from build123d import *

# Parameters (mm, degrees)
SKETCH1_R           = 7.5
BOSS_EXTRUDE1_DEPTH = 35
SKETCH2_W           = 20
SKETCH2_H           = 17.5
CUT_EXTRUDE1_DEPTH  = 50
SKETCH4_R           = 15
BOSS_EXTRUDE2_DEPTH = 30
SKETCH6_R           = 9.525
CUT_EXTRUDE2_DEPTH  = 30


with BuildPart() as part:
    # Sketch1 → Boss-Extrude1 (new body)
    with BuildSketch(Plane.XY):
        with BuildLine():
            Line((-5, 12.5), (5, 12.5))
            ThreePointArc((5, 12.5), (12.071067812, 9.571067812), (15, 2.5))
            Line((15, 2.5), (15, -12.5))
            Line((15, -12.5), (-15, -12.5))
            Line((-15, -12.5), (-15, 2.5))
            ThreePointArc((-15, 2.5), (-12.071067812, 9.571067812), (-5, 12.5))
        make_face()
        with Locations((0, 2.5)):
            Circle(SKETCH1_R, mode=Mode.SUBTRACT)
    extrude(amount=BOSS_EXTRUDE1_DEPTH)

    # Sketch2 → Cut-Extrude1 (cut)
    with BuildSketch(Plane(origin=(15, 0, 0), x_dir=(0, 0, -1), z_dir=(1, 0, 0))):
        with Locations((-17.5, 3.75)):
            Rectangle(SKETCH2_W, SKETCH2_H)
    extrude(amount=-CUT_EXTRUDE1_DEPTH, mode=Mode.SUBTRACT)

    # Sketch4 → Boss-Extrude2 (add)
    with BuildSketch(Plane.XZ.offset(12.5)):
        with Locations(Location((0, 17.5, 0), (0, 0, 180))):
            Circle(SKETCH4_R)
    extrude(amount=BOSS_EXTRUDE2_DEPTH)

    # Sketch6 → Cut-Extrude2 (cut)
    with BuildSketch(Plane.XZ.offset(42.5)):
        with Locations(Location((0, 17.5, 0), (0, 0, 270))):
            Circle(SKETCH6_R)
    extrude(amount=-CUT_EXTRUDE2_DEPTH, mode=Mode.SUBTRACT)


solid = part.part
Can you work these out from the model? Positions are in its coordinate system, mm. A direction names the side the tool comes from. Coordinates: 2 decimals unless noted, no trailing zeros. Write each loop counter-clockwise with the first axis right and the second up, starting at its lowest first coordinate (ties: lowest second). Pieces come first, ordered by that corner, then holes. Notation, with made-up numbers: (13, 61.5) -> (29, 61.5) arc R31 cw to (29, 91.5) -> close; hole circle Ø9 at (28.25, -18.5). An arc over 180 degrees is marked (long way). Answer as CSV lines item,"result".
1) Will these pins go through, and if not, where does the flat tip stop? P1, Ø6, axis at y = -32, z = 26, coming from the -X side; P2, Ø1, axis at x = -4.5, z = 22.5, coming from the +Y side; P3, Ø10, axis at x = 5.5, y = -26.5, coming from the +Z side.
Check result:
P1,"x = -13.96"
P2,"y = -5"
P3,"z = 32.49"
2) If I drill on line 1 (X direction, y = 2.5, z = 32.5); line 2 (Z direction, x = 11.5, y = 2.5); line 3 (Y direction, x = 0, z = 3.25), over which ranges is the centre line in solid material (lowest first)? Write a range as from..to.
Check result:
line 1,"-15..-7.5, 7.5..15"
line 2,"0..7.5, 27.5..35"
line 3,"-42.5..-5, 10..12.5"
3) If we section it at D-D on y = -34: Please give me the cut outline in (x, z) (3 decimals).
Check result:
outline,"circle Ø30 at (0, 17.5); hole circle Ø19.05 at (0, 17.5)"
4) If we mould it in two halves opening along X, with no side actions, what happens to faces 5 (the flat face through (15, -7, 17)), 6 (the flat face through (3.5, 9.5, 7.5)), 7 (the cylindrical face through (-5.5, 7.6, 3.7))? For each: +X half, -X half, draft (parallel to the pull), parting line (faces both ways), or undercut.
Check result:
face 5,"+X half"
face 6,"draft"
face 7,"undercut"
5) If we section it at C-C on x = 8.5: Please give me the cut outline in (y, z).
Check result:
outline,"(-42.5, 5.14) -> (-12.5, 5.14) -> (-12.5, 0) -> (11.87, 0) -> (11.87, 7.5) -> (-5, 7.5) -> (-5, 27.5) -> (11.87, 27.5) -> (11.87, 35) -> (-12.5, 35) -> (-12.5, 29.86) -> (-42.5, 29.86) -> (-42.5, 21.8) -> (-12.5, 21.8) -> (-12.5, 13.2) -> (-42.5, 13.2) -> close"
6) If we section it at A-A on y = 4: Please give me the cut outline in (x, z).
Check result:
outline,"(-14.89, 0) -> (-7.35, 0) -> (-7.35, 7.5) -> (-14.89, 7.5) -> close; (-14.89, 27.5) -> (-7.35, 27.5) -> (-7.35, 35) -> (-14.89, 35) -> close; (7.35, 0) -> (14.89, 0) -> (14.89, 7.5) -> (7.35, 7.5) -> close; (7.35, 27.5) -> (14.89, 27.5) -> (14.89, 35) -> (7.35, 35) -> close"
7) On a 3-axis mill with a long thin cutter (end or side, diameter ignored), from which of +Z, -Z, +X, -X, +Y, -Y can I reach the whole of each face in a straight line? I mean faces 1 (the flat face through (1, -12.5, 2)), 2 (the flat face through (0, -5, 18)), 3 (the flat face through (-15, -7, 17)), 4 (the cylindrical face through (-8.06, -27.29, 4.85)). Say none if no direction works.
Check result:
face 1,"-Z, -Y"
face 2,"+X, -X, +Y"
face 3,"+Z, -Z, -X, +Y, -Y"
face 4,"-Y"
8) If we section it at B-B on x = -2.75: Please give me the cut outline in (y, z).
Check result:
outline,"(-42.5, 2.75) -> (-12.5, 2.75) -> (-12.5, 0) -> (-4.48, 0) -> (-4.48, 7.5) -> (-5, 7.5) -> (-5, 27.5) -> (-4.48, 27.5) -> (-4.48, 35) -> (-12.5, 35) -> (-12.5, 32.25) -> (-42.5, 32.25) -> (-42.5, 26.62) -> (-12.5, 26.62) -> (-12.5, 8.38) -> (-42.5, 8.38) -> close; (9.48, 0) -> (12.5, 0) -> (12.5, 7.5) -> (9.48, 7.5) -> close; (9.48, 27.5) -> (12.5, 27.5) -> (12.5, 35) -> (9.48, 35) -> close"
